Solid Edge part; units mm, degrees
sketch "Sketch1" plane through (0, 0, 0) normal (0, 0, 1) x (1, 0, 0)
  line L0 (-26.9994, -20.0005) -> (26.9994, -20.0005)
  line L1 (26.9994, -20.0005) -> (26.9994, 23.0005)
  line L2 (26.9994, 23.0005) -> (-26.9994, 23.0005)
  line L3 (-26.9994, 23.0005) -> (-26.9994, -20.0005)
extrude "Protrusion1" add sketch "Sketch1" against normal blind 7
sketch "Sketch2" plane through (0, 1.5, 0) normal (0, 0, 1) x (1, 0, 0)
  line L0 (-25.9994, -20.5005) -> (25.9994, -20.5005)
  line L1 (25.9994, -20.5005) -> (25.9994, 17.5005)
  line L2 (25.9994, 17.5005) -> (-25.9994, 17.5005)
  line L3 (-25.9994, 17.5005) -> (-25.9994, -20.5005)
extrude "Extrusionsausschnitt_1" cut sketch "Sketch2" against normal blind 6
sketch "Sketch3" plane through (0, 0, -6) normal (0, 0, 1) x (1, 0, 0)
  line L0 (-26.4993, 13.4996) -> (-20.4993, 13.4996)
  line L1 (-20.4993, 13.4996) -> (-20.4993, 19.4996)
  line L2 (-20.4993, 19.4996) -> (-26.4993, 19.4996)
  line L3 (-26.4993, 19.4996) -> (-26.4993, 13.4996)
extrude "Extrusionsausprägung_2" add sketch "Sketch3" along normal blind 4.4
sketch "Sketch4" plane through (0, 0, -6) normal (0, 0, 1) x (1, 0, 0)
  line L0 (-26.4993, -19.5006) -> (-20.4993, -19.5006)
  line L1 (-20.4993, -19.5006) -> (-20.4993, -13.5006)
  line L2 (-20.4993, -13.5006) -> (-26.4993, -13.5006)
  line L3 (-26.4993, -13.5006) -> (-26.4993, -19.5006)
extrude "Protrusion2" add sketch "Sketch4" along normal blind 4.4
sketch "Sketch5" plane through (0, 0, -6) normal (0, 0, 1) x (1, 0, 0)
  line L0 (20.5006, -19.5006) -> (26.5006, -19.5006)
  line L1 (26.5006, -19.5006) -> (26.5006, -13.5006)
  line L2 (26.5006, -13.5006) -> (20.5006, -13.5006)
  line L3 (20.5006, -13.5006) -> (20.5006, -19.5006)
  line L4 (20.5006, 13.4996) -> (26.5006, 13.4996)
  line L5 (26.5006, 13.4996) -> (26.5006, 19.4996)
  line L6 (26.5006, 19.4996) -> (20.5006, 19.4996)
  line L7 (20.5006, 19.4996) -> (20.5006, 13.4996)
extrude "Extrusionsausprägung_4" add sketch "Sketch5" along normal blind 4.4
sketch "Sketch6" plane through (0, 1.5, -7) normal (0, 0, -1) x (0, -1, 0)
  circle A0 centre (-14.9996, 23.4993) radius 1.6
  circle A1 centre (18.0006, 23.4993) radius 1.6
  circle A2 centre (18.0006, -23.5006) radius 1.6
  circle A3 centre (-14.9996, -23.5006) radius 1.6
extrude "Extrusionsausschnitt_3" cut sketch "Sketch6" against normal blind 225.4763
sketch "Sketch7" plane through (0, 1.5, 0) normal (0, 0, 1) x (1, 0, 0)
  line L0 (-19.997, 17.5005) -> (20.003, 17.5005)
  line L1 (20.003, 17.5005) -> (20.003, 20.0005)
  line L2 (20.003, 20.0005) -> (-19.997, 20.0005)
  line L3 (-19.997, 20.0005) -> (-19.997, 17.5005)
  dimension "D1" = 20.003
  dimension "D2" = 20.003
extrude "Extrusionsausschnitt_4" cut sketch "Sketch7" against normal blind 2
sketch "Sketch8" plane through (0, 0, -6) normal (0, 0, 1) x (1, 0, 0)
  line L0 (17.9994, -9.5004) -> (21.9994, -9.5004)
  line L1 (21.9994, -9.5004) -> (21.9994, 10.4996)
  line L2 (21.9994, 10.4996) -> (17.9994, 10.4996)
  line L3 (17.9994, 10.4996) -> (17.9994, -9.5004)
  line L4 (9.9994, -9.5004) -> (13.9994, -9.5004)
  line L5 (13.9994, -9.5004) -> (13.9994, 10.4996)
  line L6 (13.9994, 10.4996) -> (9.9994, 10.4996)
  line L7 (9.9994, 10.4996) -> (9.9994, -9.5004)
  line L8 (1.9994, -9.5004) -> (5.9994, -9.5004)
  line L9 (5.9994, -9.5004) -> (5.9994, 10.4996)
  line L10 (5.9994, 10.4996) -> (1.9994, 10.4996)
  line L11 (1.9994, 10.4996) -> (1.9994, -9.5004)
  line L12 (-6.0006, -9.5004) -> (-2.0006, -9.5004)
  line L13 (-2.0006, -9.5004) -> (-2.0006, 10.4996)
  line L14 (-2.0006, 10.4996) -> (-6.0006, 10.4996)
  line L15 (-6.0006, 10.4996) -> (-6.0006, -9.5004)
  line L16 (-14.0006, -9.5004) -> (-10.0006, -9.5004)
  line L17 (-10.0006, -9.5004) -> (-10.0006, 10.4996)
  line L18 (-10.0006, 10.4996) -> (-14.0006, 10.4996)
  line L19 (-14.0006, 10.4996) -> (-14.0006, -9.5004)
  dimension "D1" = 21.9994
  dimension "D2" = 21.9994
extrude "Cutout1" cut sketch "Sketch8" along normal mid plane 25.2613
fillet "Verrundung_1" radius 2 20 edges at (-10.0006, 10.4996, -6.5) (-2.0006, 10.4996, -6.5) (5.9994, 10.4996, -6.5) (13.9994, 10.4996, -6.5) (21.9994, 10.4996, -6.5) (17.9994, 10.4996, -6.5) (9.9994, 10.4996, -6.5) (1.9994, 10.4996, -6.5) (-6.0006, 10.4996, -6.5) (-14.0006, 10.4996, -6.5) (-14.0006, -9.5004, -6.5) (-6.0006, -9.5004, -6.5) (1.9994, -9.5004, -6.5) (9.9994, -9.5004, -6.5) (17.9994, -9.5004, -6.5) (-10.0006, -9.5004, -6.5) (-2.0006, -9.5004, -6.5) (5.9994, -9.5004, -6.5) (13.9994, -9.5004, -6.5) (21.9994, -9.5004, -6.5)
sketch "Sketch9" plane through (0, 1.5, 0) normal (0, 0, 1) x (0, 1, 0)
  line L0 (21.3005, -40) -> (21.3005, 40)
  dimension "D1" = 21.3005
extrude "Extrusionsausschnitt_6" cut sketch "Sketch9" along normal mid plane 56.5078 material side at (0, 22.8505, 0)
sketch "Sketch10" plane through (0, 1.4, 0) normal (0, 0, 1) x (1, 0, 0)
  line L0 (-26.3, -20.7) -> (26.3, -20.7)
  line L1 (26.3, -20.7) -> (26.3, 17.9)
  line L2 (26.3, 17.9) -> (-26.3, 17.9)
  line L3 (-26.3, 17.9) -> (-26.3, -20.7)
  dimension "D1" = 26.3
  dimension "D2" = 26.3
extrude "Extrusionsausschnitt_7" cut sketch "Sketch10" against normal blind 2
sketch "Sketch11" plane through (0, 22.8005, -3.5) normal (0, 1, 0) x (1, 0, 0)
  line L0 (-26.9994, -3.5) -> (26.9994, -3.5)
  line L1 (26.9994, -3.5) -> (26.9994, 3.5)
  line L2 (26.9994, 3.5) -> (-26.9994, 3.5)
  line L3 (-26.9994, 3.5) -> (-26.9994, -3.5)
extrude "Protrusion3" add sketch "Sketch11" along normal blind 0.5
chamfer "Chamfer1" distance 1.75 angle 45 1 edges at (23.5006, 18.0996, -7)
chamfer "Fase_3" distance 1.75 angle 45 3 edges at (23.5006, -14.9006, -7) (-23.4993, -14.9006, -7) (-23.4993, 18.0996, -7)
The model under review builds one solid part; all positions refer to its coordinate system, in mm. A direction names the side the tool comes from. Round coordinates to 2 decimals unless told otherwise and drop trailing zeros. Write each loop counter-clockwise with the first axis right and the second up, starting at its lowest first coordinate (ties: lowest second). Pieces come first, ordered by that corner, then holes. Notation, with made-up numbers: (-9, 60.5) - (10, 60.5) arc R29 cw to (10, 92.5) - close; hole circle Ø2 at (41, 3). An arc over 180 degrees is marked (long way). Answer as CSV lines item,"result". Start each with the question number.
(1) We need section C-C on y = -12.5. State the section outline as (x, z) points.
(2) We need section B-B on z = -1.25. State the section outline as (x, y) points.
(3) Draft analysis for pull direction Y (two halves, no side actions). For faces 1 (the cylindrical face through (18.57, 9.9, -6.51)), 2 (the flat face through (-26.999, 2, -3)), 3 (the flat face through (-26.3, 0, -1)), state which applies: pulls with the +Y half, pulls with the -Y half, needs draft (parallel to the pull), parting line crosses it, or undercut.
(4) We need section A-A on y = 3.5. Give the number of separate pieces and of enclosed holes in the cut face, plus the area to 3 significant figures.
(5) We need section D-D on x = -11. State the section outline as (y, z) points.
(6) To check wall thickness, follow line 1 (X direction, y = 5.5, z = -6.5); line 2 (Y direction, x = 16.5, z = -5.5); line 3 (Y direction, x = -24, z = -0.25). State the ranges of each line that lie inside material, in increasing order.
(7) For pin 1 Ø8 at (x, y) = (14.5, 12.5) entering from +Z, flat-tipped, find the tip position at first contact; note if it passes through.
(8) For faces 4 (the flat face through (-25.999, 0, -4)), 5 (the cylindrical face through (-5.43, 9.9, -6.51)), list the 3-axis set-ups (+Z, -Z, +X, -X, +Y, -Y) from which the entire face can be reached by the end or side of a thin tool; tool diameter is ignored.
Worked answers:
1,outline,"(-27, -7) - (27, -7) - (27, 0) - (26.3, 0) - (26.3, -2) - (26, -2) - (26, -6) - (-26, -6) - (-26, -2) - (-26.3, -2) - (-26.3, 0) - (-27, 0) - close"
2,outline,"(-27, -20) - (27, -20) - (27, 23.3) - (-27, 23.3) - close; hole (-26.3, -19.3) - (26.3, -19.3) - (26.3, 19.3) - (20, 19.3) - (20, 21.5) - (-20, 21.5) - (-20, 19.3) - (-26.3, 19.3) - close"
3,face 1,"undercut"
3,face 2,"needs draft"
3,face 3,"undercut"
4,separate pieces,"6"
4,enclosed holes,"0"
4,area,"44.8 mm²"
5,outline,"(-20, -7) - (-9.23, -7) - (-9.23, -6) - (-19, -6) - (-19, -2) - (-19.3, -2) - (-19.3, 0) - (-20, 0) - close; (10.23, -7) - (23.3, -7) - (23.3, 0) - (21.5, 0) - (21.5, -2) - (19, -2) - (19, -6) - (10.23, -6) - close"
6,line 1,"-27 to -14, -10 to -6, -2 to 2, 6 to 10, 14 to 18, 22 to 27"
6,line 2,"-20 to -19, 19 to 23.3"
6,line 3,"-20 to -19.3, 19.3 to 23.3"
7,pin 1,"z = -6"
8,face 4,"+Z"
8,face 5,"+Z, -Z"
